```python
from build123d import *

# Parameters (mm, degrees)
F1_DEPTH = 20
F3_R     = 1.65
F4_DEPTH = 25
F2_R     = 1.65
F5_DEPTH = 25


with BuildPart() as f1:
    # F0 (on Top) → F1 (new body)
    with BuildSketch(Plane.XY):
        with BuildLine():
            ThreePointArc((-13.1, 0), (0, 13.1), (13.1, 0))
            Line((13.1, 0), (20.6, 0))
            Line((20.6, 0), (20.6, 2))
            Line((20.6, 2), (14.966964, 2))
            ThreePointArc((14.966964, 2), (0, 15.1), (-14.966964, 2))
            Line((-14.966964, 2), (-20.6, 2))
            Line((-20.6, 2), (-20.6, 0))
            Line((-20.6, 0), (-13.1, 0))
        make_face()
    extrude(amount=F1_DEPTH)

    # F3 (on face) → F4 (cut)
    with BuildSketch(Plane(origin=(0, 2, 0), x_dir=(-1, 0, 0), z_dir=(0, 1, 0))):
        with Locations((17.783482, 16.35)):
            Circle(F3_R)
        with Locations((17.783482, 3.65)):
            Circle(F3_R)
    extrude(amount=-F4_DEPTH, mode=Mode.SUBTRACT)

    # F2 (on face) → F5 (cut)
    with BuildSketch(Plane(origin=(0, 2, 0), x_dir=(-1, 0, 0), z_dir=(0, 1, 0))):
        with Locations((-17.783482, 16.35)):
            Circle(F2_R)
        with Locations((-17.783482, 3.65)):
            Circle(F2_R)
    extrude(amount=-F5_DEPTH, mode=Mode.SUBTRACT)


solid = f1.part
```
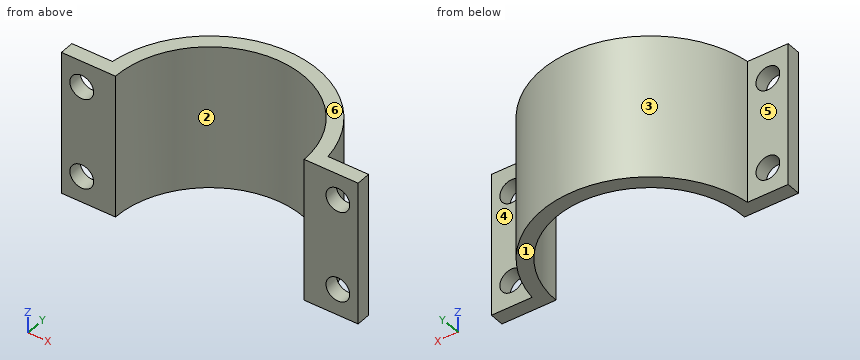
Could you check a few things on this model? Use its own coordinates, in mm. Face numbers are marked on the shaded views. A direction names the side the tool comes from. Round coordinates to 2 decimals unless told otherwise and drop trailing zeros. Loops run counter-clockwise (first coordinate to the right, second up) from the corner with the lowest first, then second, coordinate; pieces in that order, holes last. Notation, with made-up numbers: (12, 27) -> (42, 27) arc R34 cw to (42, 63) -> close; hole circle Ø7 at (64.5, -33.75). An arc over 180 degrees is marked (long way). Put each result on its own line as item: value.
Q1. For pin 1 Ø4 at (y, z) = (11.5, 13) entering from +X; pin 2 Ø4 at (x, z) = (-17.78, 3.65) entering from -Y; pin 3 Ø4 at (y, z) = (8, 3.5) entering from -X; pin 4 Ø8 at (y, z) = (8.5, 2.5) entering from -X, each with a flat end and sliding along its axis, tell me the tip position at first contact or that it passes through.
Checks:
pin 1: x = 11.74
pin 2: y = 0
pin 3: x = -13.86
pin 4: x = -14.41
Q2. I want a section at C-C on z = 11.25. Write out the boundary of the cut face in (x, y), and give its area (3 significant figures).
Checks:
outline: (-20.6, 0) -> (-13.1, 0) arc R13.1 cw to (13.1, 0) -> (20.6, 0) -> (20.6, 2) -> (14.97, 2) arc R15.1 ccw to (-14.97, 2) -> (-20.6, 2) -> close
area: 111 mm2
Q3. Which directions (+Z, -Z, +X, -X, +Y, -Y) give clear straight access to the entire face, cutting with the end or side of a thin tool? Please do the marked faces 4, 5 and 6.
Checks:
face 4: +Z, -Z, +X, +Y
face 5: +Z, -Z, -X, +Y
face 6: +Z, +X, -X, +Y, -Y
Q4. I want a section at A-A on z = 16.35. Write out the boundary of the cut face in (x, y).
Checks:
outline: (-20.6, 0) -> (-19.43, 0) -> (-19.43, 2) -> (-20.6, 2) -> close; (-16.13, 0) -> (-13.1, 0) arc R13.1 cw to (13.1, 0) -> (16.13, 0) -> (16.13, 2) -> (14.97, 2) arc R15.1 ccw to (-14.97, 2) -> (-16.13, 2) -> close; (19.43, 0) -> (20.6, 0) -> (20.6, 2) -> (19.43, 2) -> close
Q5. I want a section at B-B on y = 7. Write out the boundary of the cut face in (x, z), and give its area (3 significant figures).
Checks:
outline: (-13.38, 0) -> (-11.07, 0) -> (-11.07, 20) -> (-13.38, 20) -> close; (11.07, 0) -> (13.38, 0) -> (13.38, 20) -> (11.07, 20) -> close
area: 92.3 mm2
Q6. Thinking about a two-plate mould opening in X: for the marked faces 1, 2 and 3, which applies, pulls with the +X half, pulls with the -X half, needs draft (parallel to the pull), parting line crosses it, or undercut?
Checks:
face 1: needs draft
face 2: undercut
face 3: parting line crosses it
Q7. I want a section at D-D on x = 0. Write out the boundary of the cut face in (y, z), and give its area (3 significant figures).
Checks:
outline: (13.1, 0) -> (15.1, 0) -> (15.1, 20) -> (13.1, 20) -> close
area: 40.0 mm2
Q8. Please list where these lines run through material, in increasing order: line 1 (Y direction, x = 0.5, z = 10); line 2 (X direction, y = 7, z = 4); line 3 (Y direction, x = -17, z = 18.75). Write a range as from..to.
Checks:
line 1: 13.09..15.09
line 2: -13.38..-11.07, 11.07..13.38
line 3: 0..2
